Geometry check sheet. Reference: the model listing, model coordinates, mm. A direction names the side the tool comes from. Coordinates: 2 decimals unless noted, no trailing zeros. Write each loop counter-clockwise with the first axis right and the second up, starting at its lowest first coordinate (ties: lowest second). Pieces come first, ordered by that corner, then holes. Notation, with made-up numbers: (40, 68) -> (74, 68) arc R24 cw to (74, 101) -> close; hole circle Ø6 at (-19.5, -38.75). An arc over 180 degrees is marked (long way). One line per question, with ' | ' between items.
from build123d import *

# Parameters (mm, degrees)
SKETCH3_W           = 50.8
SKETCH3_H           = 50.8
BOSS_EXTRUDE1_DEPTH = 1.27
CUT_EXTRUDE1_REACH  = 3.27
SKETCH4_R           = 1.0999978
SKETCH5_W           = 17.78
SKETCH5_H           = 35.56
SKETCH5_W_2         = 13.97
SKETCH5_H_2         = 34.29
BOSS_EXTRUDE2_DEPTH = 7.62
SKETCH6_W           = 14.8000212
SKETCH6_H           = 14.2999968
BOSS_EXTRUDE3_DEPTH = 5.334
BOSS_EXTRUDE4_DEPTH = 12.7
SKETCH8_W           = 11.43
SKETCH8_H           = 15.24
SKETCH8_H_2         = 10.16
BOSS_EXTRUDE5_DEPTH = 6.35
SKETCH9_W           = 3.81
SKETCH9_H           = 10.16
BOSS_EXTRUDE6_DEPTH = 12.7
SKETCH10_W          = 0.635
SKETCH10_H          = 10.16
BOSS_EXTRUDE7_DEPTH = 19.05


with BuildPart() as part:
    # Sketch3 → Boss-Extrude1 (new body)
    with BuildSketch(Plane(origin=(0, 0, 0), x_dir=(1, 0, 0), z_dir=(0, 1, 0))):
        with Locations((25.4, 25.4)):
            Rectangle(SKETCH3_W, SKETCH3_H)
    extrude(amount=BOSS_EXTRUDE1_DEPTH)

    # Sketch4 → Cut-Extrude1 (cut, up to next)
    with BuildSketch(Plane(origin=(0, 0, 0), x_dir=(1, 0, 0), z_dir=(0, 1, 0)), mode=Mode.PRIVATE) as cut_extrude1_sk1:
        with Locations((1.905, 48.895)):
            Circle(SKETCH4_R)
    cut_extrude1_tool1 = extrude(cut_extrude1_sk1.sketch, amount=CUT_EXTRUDE1_REACH, mode=Mode.PRIVATE) & part.part
    add(cut_extrude1_tool1.solids().sort_by_distance((1.905, 0, -48.895))[0], mode=Mode.SUBTRACT)
    # Sketch4 → Cut-Extrude1 (cut, up to next)
    with BuildSketch(Plane(origin=(0, 0, 0), x_dir=(1, 0, 0), z_dir=(0, 1, 0)), mode=Mode.PRIVATE) as cut_extrude1_sk2:
        with Locations((48.895, 48.895)):
            Circle(SKETCH4_R)
    cut_extrude1_tool2 = extrude(cut_extrude1_sk2.sketch, amount=CUT_EXTRUDE1_REACH, mode=Mode.PRIVATE) & part.part
    add(cut_extrude1_tool2.solids().sort_by_distance((48.895, 0, -48.895))[0], mode=Mode.SUBTRACT)
    # Sketch4 → Cut-Extrude1 (cut, up to next)
    with BuildSketch(Plane(origin=(0, 0, 0), x_dir=(1, 0, 0), z_dir=(0, 1, 0)), mode=Mode.PRIVATE) as cut_extrude1_sk3:
        with Locations((48.895, 1.905)):
            Circle(SKETCH4_R)
    cut_extrude1_tool3 = extrude(cut_extrude1_sk3.sketch, amount=CUT_EXTRUDE1_REACH, mode=Mode.PRIVATE) & part.part
    add(cut_extrude1_tool3.solids().sort_by_distance((48.895, 0, -1.905))[0], mode=Mode.SUBTRACT)
    # Sketch4 → Cut-Extrude1 (cut, up to next)
    with BuildSketch(Plane(origin=(0, 0, 0), x_dir=(1, 0, 0), z_dir=(0, 1, 0)), mode=Mode.PRIVATE) as cut_extrude1_sk4:
        with Locations((1.905, 1.905)):
            Circle(SKETCH4_R)
    cut_extrude1_tool4 = extrude(cut_extrude1_sk4.sketch, amount=CUT_EXTRUDE1_REACH, mode=Mode.PRIVATE) & part.part
    add(cut_extrude1_tool4.solids().sort_by_distance((1.905, 0, -1.905))[0], mode=Mode.SUBTRACT)

    # Sketch5 → Boss-Extrude2 (add)
    with BuildSketch(Plane(origin=(0, 1.27, 0), x_dir=(1, 0, 0), z_dir=(0, 1, 0))):
        with Locations((34.29, 19.05)):
            Rectangle(SKETCH5_W, SKETCH5_H)
        with Locations((17.78, 18.415)):
            Rectangle(SKETCH5_W_2, SKETCH5_H_2)
    extrude(amount=BOSS_EXTRUDE2_DEPTH)

    # Sketch6 → Boss-Extrude3 (add)
    with BuildSketch(Plane(origin=(0, 1.27, 0), x_dir=(1, 0, 0), z_dir=(0, 1, 0))):
        with Locations((39.37, 46.219999)):
            Rectangle(SKETCH6_W, SKETCH6_H)
    extrude(amount=BOSS_EXTRUDE3_DEPTH)

    # Sketch7 → Boss-Extrude4 (add)
    with BuildSketch(Plane(origin=(0, 1.27, 0), x_dir=(1, 0, 0), z_dir=(0, 1, 0))):
        Polygon((4.390009, 53.2400002), (13.389991, 53.2400002), (13.389991, 50.340006), (13.389991, 39.640002), (4.390009, 39.640002), align=None)
    extrude(amount=BOSS_EXTRUDE4_DEPTH)

    # Sketch8 → Boss-Extrude5 (add)
    with BuildSketch(Plane(origin=(0, 1.27, 0), x_dir=(1, 0, 0), z_dir=(0, 1, 0))):
        with Locations((0.635, 11.43)):
            Rectangle(SKETCH8_W, SKETCH8_H)
        with Locations((0.635, 25.4)):
            Rectangle(SKETCH8_W, SKETCH8_H_2)
        with Locations((52.705, 27.94)):
            Rectangle(SKETCH8_W, SKETCH8_H)
        with Locations((52.705, 11.43)):
            Rectangle(SKETCH8_W, SKETCH8_H)
    extrude(amount=BOSS_EXTRUDE5_DEPTH)

    # Sketch9 → Boss-Extrude6 (add)
    with BuildSketch(Plane(origin=(0, 1.27, 0), x_dir=(1, 0, 0), z_dir=(0, 1, 0))):
        with Locations((21.59, 43.18)):
            Rectangle(SKETCH9_W, SKETCH9_H)
        with Locations((16.51, 43.18)):
            Rectangle(SKETCH9_W, SKETCH9_H)
    extrude(amount=BOSS_EXTRUDE6_DEPTH)

    # Sketch10 → Boss-Extrude7 (add)
    with BuildSketch(Plane(origin=(0, 1.27, 0), x_dir=(1, 0, 0), z_dir=(0, 1, 0))):
        with Locations((19.3675, 43.18)):
            Rectangle(SKETCH10_W, SKETCH10_H)
        with Locations((14.2875, 43.18)):
            Rectangle(SKETCH10_W, SKETCH10_H)
    extrude(amount=BOSS_EXTRUDE7_DEPTH)


solid = part.part
1. Cross-section at C-C on x = 49. Record the boundary of the cut face in (y, z), and give its area (3 significant figures).
Worked answers:
outline: (0, -50.8) -> (1.27, -50.8) -> (1.27, -49.99) -> (0, -49.99) -> close; (0, -47.8) -> (1.27, -47.8) -> (1.27, -35.56) -> (7.62, -35.56) -> (7.62, -20.32) -> (1.27, -20.32) -> (1.27, -19.05) -> (7.62, -19.05) -> (7.62, -3.81) -> (1.27, -3.81) -> (1.27, -3) -> (0, -3) -> close; (0, -0.81) -> (1.27, -0.81) -> (1.27, 0) -> (0, 0) -> close | area: 253 mm²
2. Cross-section at D-D on z = -16. Record the boundary of the cut face in (x, y) (3 decimals).
Worked answers:
outline: (-5.08, 1.27) -> (0, 1.27) -> (0, 0) -> (50.8, 0) -> (50.8, 1.27) -> (58.42, 1.27) -> (58.42, 7.62) -> (46.99, 7.62) -> (46.99, 1.27) -> (43.18, 1.27) -> (43.18, 8.89) -> (25.4, 8.89) -> (25.4, 1.27) -> (24.765, 1.27) -> (24.765, 8.89) -> (10.795, 8.89) -> (10.795, 1.27) -> (6.35, 1.27) -> (6.35, 7.62) -> (-5.08, 7.62) -> close
3. Material ranges on line 1 (X direction, y = 3.75, z = -28) (3 decimals); line 2 (Z direction, x = 5, y = 5.25); line 3 (Z direction, x = 17, y = 1.75), recorded low to high. Write a range as from..to.
Worked answers:
line 1: -5.08..6.35, 10.795..24.765, 25.4..43.18, 46.99..58.42 | line 2: -53.24..-39.64, -30.48..-20.32, -19.05..-3.81 | line 3: -48.26..-38.1, -35.56..-1.27
4. Mould release check, pull along Z, two halves, no side actions. Record for faces 1 (the face through (18, 5, -1.27)), 2 (the face through (24.765, 5, -18)), 3 (the face through (18, 5, -35.56)): released by +Z, released by -Z, zero draft, split by the parting line, or undercut.
Worked answers:
face 1: released by +Z | face 2: zero draft | face 3: undercut
5. Go/stop test with flat-tipped pins: P1, Ø1, axis at x = 31.5, y = 1, coming from the -Z side; P2, Ø5, axis at x = 46.5, z = -9, coming from the +Y side; P3, Ø4, axis at x = 20.5, y = 7, coming from the +Z side; P4, Ø2, axis at x = 48.895, z = -48.895, coming from the -Y side. Record where each tip stops, or that it passes through.
Worked answers:
P1: z = -50.8 | P2: y = 7.62 | P3: z = -1.27 | P4: through
6. Cross-section at A-A on y = 10.5. Record the boundary of the cut face in (x, z) (3 decimals), and give its area (3 significant figures).
Worked answers:
outline: (4.39, -53.24) -> (13.39, -53.24) -> (13.39, -39.64) -> (4.39, -39.64) -> close; (13.97, -48.26) -> (18.415, -48.26) -> (18.415, -38.1) -> (13.97, -38.1) -> close; (19.05, -48.26) -> (23.495, -48.26) -> (23.495, -38.1) -> (19.05, -38.1) -> close | area: 213 mm²
7. Cross-section at B-B on y = 16.5. Record the boundary of the cut face in (x, z) (3 decimals).
Worked answers:
outline: (13.97, -48.26) -> (14.605, -48.26) -> (14.605, -38.1) -> (13.97, -38.1) -> close; (19.05, -48.26) -> (19.685, -48.26) -> (19.685, -38.1) -> (19.05, -38.1) -> close
8. Tool access check on faces 4 (the face through (25.4, 5, -19)), 5 (the face through (31.97, 4, -46)), 6 (the face through (9, 13.97, -47)), 7 (the face through (18, 8.89, -19)), 8 (the face through (10.795, 5, -18)). Record the directions out of +Z, -Z, +X, -X, +Y, -Y that give a thin tool (end or side, any length) a straight path to the whole face; none if there is none.
Worked answers:
face 4: +Z, -Z, +Y | face 5: -Z, +Y | face 6: +Z, -Z, -X, +Y | face 7: +Z, +X, -X, +Y | face 8: +Z, +Y
